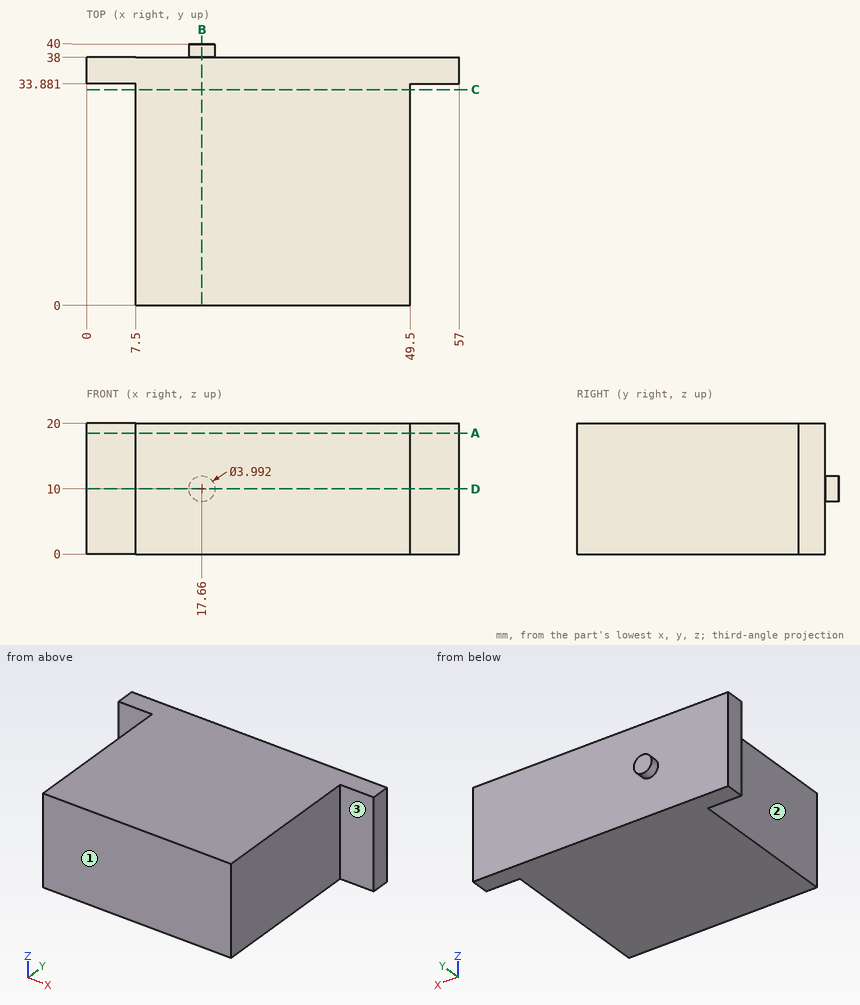
Answer from the drawing. Dimensions are ordinates in mm from the lowest x, y and z of the part. A direction names the side the tool comes from. Coordinates: 2 decimals unless noted, no trailing zeros. Loops run counter-clockwise (first coordinate to the right, second up) from the corner with the lowest first, then second, coordinate; pieces in that order, holes last. Notation, with made-up numbers: (89.25, 53) -> (144.25, 53) arc R24 cw to (144.25, 92) -> close; hole circle Ø2 at (18, -3.5). An arc over 180 degrees is marked (long way). Answer as CSV lines item,"result".
Q1. A tool of negligible diameter and unlimited length cuts with its end or side. For the marked faces 1, 2 and 3, from which of +Z, -Z, +X, -X, +Y, -Y can it reach the whole face along a straight path? Write none if from no direction.
Findings:
face 1,"+Z, -Z, +X, -X, -Y"
face 2,"+Z, -Z, -X, -Y"
face 3,"+Z, -Z, +X, -Y"
Q2. Find the intervals of material crossed by probe 1 along X at (y, z) = (21, 17.75); probe 2 along Y at (x, z) = (48, 11.25); probe 3 along Y at (x, z) = (50, 16.5), in increasing order.
Findings:
probe 1,"x = 7.5 to 49.5"
probe 2,"y = 0 to 38"
probe 3,"y = 33.88 to 38"
Q3. The part is cut by section B-B on x = 17.66. Write down the section's boundary in (y, z), and give its area (3 significant figures).
Findings:
outline,"(0, 0) -> (38, 0) -> (38, 8) -> (40, 8) -> (40, 12) -> (38, 12) -> (38, 20) -> (0, 20) -> close"
area,"768 mm²"
Q4. The part is cut by section D-D on z = 10. Write down the section's boundary in (x, y), and give its area (3 significant figures).
Findings:
outline,"(0, 33.88) -> (7.5, 33.88) -> (7.5, 0) -> (49.5, 0) -> (49.5, 33.88) -> (57, 33.88) -> (57, 38) -> (19.66, 38) -> (19.66, 40) -> (15.66, 40) -> (15.66, 38) -> (0, 38) -> close"
area,"1,670 mm²"
Q5. The part is cut by section C-C on y = 33. Write down the section's boundary in (x, z), and give its area (3 significant figures).
Findings:
outline,"(7.5, 0) -> (49.5, 0) -> (49.5, 20) -> (7.5, 20) -> close"
area,"840 mm²"
Q6. The part is cut by section A-A on z = 18.5. Write down the section's boundary in (x, y), and give its area (3 significant figures).
Findings:
outline,"(0, 33.88) -> (7.5, 33.88) -> (7.5, 0) -> (49.5, 0) -> (49.5, 33.88) -> (57, 33.88) -> (57, 38) -> (0, 38) -> close"
area,"1,660 mm²"
Q7. Each of these flat-tipped pins is pushed along its axis until it touches: pin 1 (10 mm diameter, centred on y = 6, z = 18, fed in from -X); pin 2 (1 mm diameter, centred on x = 46, z = 16.5, fed in from +Y); pin 3 (10 mm diameter, centred on y = 16, z = 17.5, fed in from +X). Where does it stop, or does it pass through?
Findings:
pin 1,"stops at x = 7.5"
pin 2,"stops at y = 38"
pin 3,"stops at x = 49.5"
